Read the model definition and answer for the solid it produces. Units are mm, in the model's axes. Face numbers are marked on the shaded views. A direction names the side the tool comes from. Coordinates: 2 decimals unless noted, no trailing zeros. Loops run counter-clockwise (first coordinate to the right, second up) from the corner with the lowest first, then second, coordinate; pieces in that order, holes last. Notation, with made-up numbers: (65, 43) -> (72, 43) arc R14 cw to (72, 47) -> close; hole circle Ø10 at (-16, -29). An arc over 180 degrees is marked (long way). Answer as a JSON object with one key per item and string values. Group by question number.
1) Flat-ended cylindrical pins translate along their axes: P1, Ø4, axis at x = -5, z = 0.5, coming from the -Y side; P2, Ø5, axis at x = 12.6, z = 0, coming from the +Y side; P3, Ø3, axis at y = -4.5, z = 9, coming from the +X side; P4, Ø2, axis at y = -1.5, z = -6.5, coming from the +X side. Find the tip coordinate at first contact, or state that the pin passes through.
2) Section B-B, the plane y = -4.75 is taken. Give the vertices of the cut face in (x, z), plus the area to 3 significant figures.
3) Determine the mould class of the marked faces 1 and 2 for opening direction X: released by +X, released by -X, zero draft, split by the parting line, or undercut.
4) Section C-C, the plane y = -2 is taken. Give the vertices of the cut face in (x, z) (3 decimals), plus the area to 3 significant figures.
5) Consider probe 1 along X at (y, z) = (-3.25, -2.5); probe 2 along X at (y, z) = (-3.75, -2.75); probe 3 along Y at (x, z) = (6, -7.75). Determine where each line is inside the solid, lowest interval first. Write a range as [from, to].
6) Which of the six approach directions +Z, -Z, +X, -X, +Y, -Y give full straight-line access (tool end or side, diameter ignored) to the marked faces 3 and 4?
7) Section D-D, the plane x = -10 is taken. Give the vertices of the cut face in (y, z), plus the area to 3 significant figures.
8) Section A-A, the plane z = 2.25 is taken. Give the vertices of the cut face in (x, y).
from build123d import *

# Parameters (mm, degrees)
F0_R     = 2.733615219
F0_R_2   = 3
F1_DEPTH = 4
F2_R     = 6.1140658309
F2_R_2   = 3
F3_DEPTH = 3


with BuildPart() as f1:
    # F0 (on Front) → F1 (new body)
    with BuildSketch(Plane.XZ):
        with BuildLine():
            ThreePointArc((-20.9291024725, 3.9184624391), (-25.5731023406, 11.0220372274), (-33.4257613217, 14.2412384443))
            Line((-33.4257613217, 14.2412384443), (-33.8473095456, 14.2720264872))
            ThreePointArc((-33.8473095456, 14.2720264872), (-48.8397789722, 1.9540051753), (-37.7431354391, -13.9636671057))
            Line((-37.7431354391, -13.9636671057), (-39.344081143, -3.2314471709))
            ThreePointArc((-39.344081143, -3.2314471709), (-38.4309864787, 1.2020468529), (-34.8697970186, 3.9962445472))
            ThreePointArc((-34.8697970186, 3.9962445472), (-31.8036791498, 4.3867256224), (-28.7131243857, 4.4317312401))
            ThreePointArc((-28.7131243857, 4.4317312401), (-24.811331448, 4.3234463104), (-20.9291024725, 3.9184624391))
        make_face()
        with Locations((-40.4446981847, 6.723803468)):
            Circle(F0_R, mode=Mode.SUBTRACT)
        with BuildLine():
            ThreePointArc((5.1346311332, -7.8763348549), (2.6715056736, 4.3819848217), (13.3886933806, 10.8221149428))
            Line((13.3886933806, 10.8221149428), (-33.4257613217, 14.2412384443))
            ThreePointArc((-33.4257613217, 14.2412384443), (-25.5731023406, 11.0220372274), (-20.9291024725, 3.9184624391))
            ThreePointArc((-20.9291024725, 3.9184624391), (-7.0573737231, -0.1230384341), (5.1346311332, -7.8763348549))
        make_face()
        with BuildLine():
            ThreePointArc((13.4524496929, -10.8172695714), (20.5673366745, -7.3645945031), (23.4492335658, 0))
            ThreePointArc((23.4492335658, 0), (20.5456038096, 7.3880417001), (13.3886933806, 10.8221149428))
            ThreePointArc((13.3886933806, 10.8221149428), (2.6715056736, 4.3819848217), (5.1346311332, -7.8763348549))
            ThreePointArc((5.1346311332, -7.8763348549), (5.2764555881, -8.0083454106), (5.4206145263, -8.137802598))
            ThreePointArc((5.4206145263, -8.137802598), (5.901055097, -8.5116123819), (6.3773961579, -8.8906322891))
            ThreePointArc((6.3773961579, -8.8906322891), (9.0400253079, -10.2509332643), (11.972827524, -10.8328988092))
            Line((11.972827524, -10.8328988092), (13.4524496929, -10.8172695714))
        make_face()
        with Locations((12.5982933263, 0)):
            Circle(F0_R_2, mode=Mode.SUBTRACT)
    extrude(amount=F1_DEPTH)

    # F2 (on face) → F3 (join)
    with BuildSketch(Plane.XZ.offset(4)):
        with Locations((12.5982933263, 0)):
            Circle(F2_R)
        with Locations((12.5982933263, 0)):
            Circle(F2_R_2, mode=Mode.SUBTRACT)
    extrude(amount=F3_DEPTH)


solid = f1.part
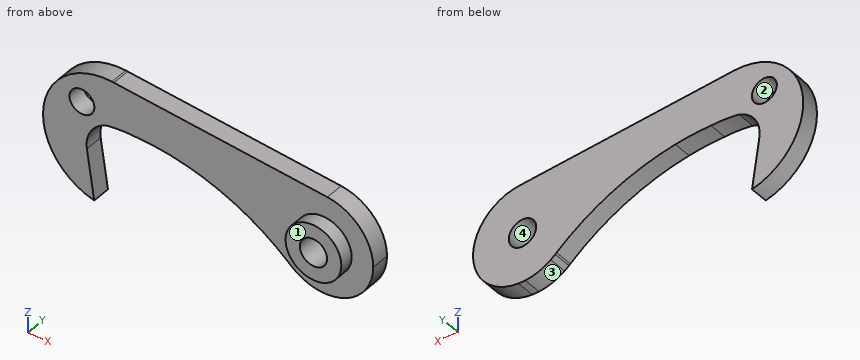
Determined:
{
 "1": {"P1": "y = -4", "P2": "through", "P3": "x = 20.36", "P4": "x = 21.95"},
 "2": {"outline": "circle Ø12.23 at (12.6, 0); hole circle Ø6 at (12.6, 0)", "area": "89.2 mm²"},
 "3": {"face 1": "zero draft", "face 2": "undercut"},
 "4": {"outline": "(-39.344, -3.231) arc R6.579 cw to (-34.87, 3.996) arc R27.584 cw to (-28.713, 4.432) arc R51.239 cw to (5.135, -7.876) arc R10.851 ccw to (5.421, -8.138) arc R55.894 cw to (6.377, -8.891) arc R10.851 ccw to (11.973, -10.833) -> (13.452, -10.817) arc R10.851 ccw to (13.389, 10.822) -> (-33.847, 14.272) arc R14.296 ccw to (-37.743, -13.964) -> close; hole circle Ø5.467 at (-40.445, 6.724); hole circle Ø6 at (12.598, 0)", "area": "1,010 mm²"},
 "5": {"probe 1": "[-48.75, -39.41], [-2.44, 10.94], [14.26, 23.16]", "probe 2": "[-48.71, -39.4], [-2.02, 11.4], [13.8, 23.09]", "probe 3": "[-4, 0]"},
 "6": {"face 3": "-Z, +Y, -Y", "face 4": "+Y, -Y"},
 "7": {"outline": "(-4, 1.1) -> (0, 1.1) -> (0, 12.53) -> (-4, 12.53) -> close", "area": "45.7 mm²"},
 "8": {"outline": "(-48.8, -4) -> (-37.63, -4) -> (-37.63, 0) -> (-48.8, 0) -> close; (-13.38, -4) -> (6.91, -4) -> (6.91, -7) -> (10.61, -7) -> (10.61, 0) -> (-13.38, 0) -> close; (14.58, -7) -> (18.28, -7) -> (18.28, -4) -> (23.21, -4) -> (23.21, 0) -> (14.58, 0) -> close"}
}
